Autodesk Fusion 360 part; units mm, degrees
sketch "Sketch1" plane through (0, 0, 0) normal (0, 0, 1) x (1, 0, 0) in component "Airfoil structure"
  spline S0 degree 5 poles (152.8506, 9.5306) (153.6754, 9.3537) (155.1958, 9.0287) (157.0885, 8.6275) (158.936, 8.2427) (160.6637, 7.8881) (162.4454, 7.5151) (164.8303, 6.998) (168.0437, 6.2836) (171.9513, 5.3996) (176.2204, 4.4167) (180.4193, 3.4264) (184.1364, 2.5129) (187.0894, 1.7283) (189.2467, 1.0645) (190.9412, 0.4268) (192.3181, -0.1665) (193.5665, -0.7111) (194.5238, -1.126) (195.0337, -1.3464) knots 0 0 0 0 0 0 0.066667 0.133333 0.2 0.266667 0.333333 0.4 0.466667 0.533333 0.6 0.666667 0.733333 0.8 0.866667 0.933333 1 1 1 1 1 1
  line L0 (148.4907, 10.4656) -> (157.2105, 8.5955)
  line L1 (191.9852, -0.0289) -> (198.0822, -2.6639)
  circle A0 centre (33.1388, 9.1296) radius 4.765
  circle A1 centre (116.1615, 7.0362) radius 3.175
  spline S1 degree 5 poles (-3.081, -1.3464) (-3.6016, -1.2536) (-4.5414, -1.0763) (-5.6463, -0.8353) (-6.5938, -0.5669) (-7.329, -0.2953) (-8.0513, 0.0089) (-9.0194, 0.5707) (-10.0683, 1.7874) (-10.9642, 3.2518) (-11.5103, 4.4866) (-11.5777, 5.0951) (-11.407, 5.643) (-11.0112, 6.6067) (-10.1307, 7.993) (-8.6022, 9.6431) (-6.4035, 11.272) (-4.1965, 12.5715) (-2.7349, 13.4061) (-1.8316, 13.8946) (-1.0216, 14.2664) (0.0955, 14.6934) (1.459, 15.1916) (2.6392, 15.6173) (3.2971, 15.8534) knots 0 0 0 0 0 0 0.05 0.1 0.15 0.2 0.25 0.3 0.35 0.4 0.45 0.5 0.55 0.6 0.65 0.7 0.75 0.8 0.85 0.9 0.95 1 1 1 1 1 1
  line L2 (0.5703, -1.9971) -> (-6.7323, -0.6957)
  line L3 (-0.0118, 14.6656) -> (6.606, 17.0412)
  line L4 (-8.4792, 9.8153) -> (-3.9569, 12.8132)
  line L5 (-11.5034, 4.2257) -> (-11.5345, 5.6935)
  line L6 (-7.2174, -0.5359) -> (-9.7443, 1.1286)
  line L7 (19.5688, 19.3646) -> (90.5688, 19.3646)
  spline S2 degree 5 poles (93.5688, 19.3646) (93.8188, 19.3387) (94.2829, 19.2905) (94.8714, 19.229) (95.4658, 19.1659) (96.0263, 19.1049) (96.567, 19.0445) (97.2368, 18.9678) (98.1315, 18.8622) (99.313, 18.7173) (100.8214, 18.5245) (102.3118, 18.3263) (103.5973, 18.1504) (104.53, 18.0207) (105.0153, 17.9528) knots 0 0 0 0 0 0 0.1 0.2 0.3 0.4 0.5 0.6 0.7 0.8 0.9 1 1 1 1 1 1
  line L8 (92.266, 19.4996) -> (94.8715, 19.2297)
  line L9 (103.6448, 18.1447) -> (106.3858, 17.761)
  spline S3 degree 5 poles (6.5765, 16.943) (6.9079, 17.0449) (7.5374, 17.2364) (8.3817, 17.4868) (9.3156, 17.7508) (10.2084, 17.9865) (10.8922, 18.156) (11.4504, 18.29) (11.9864, 18.4184) (12.6265, 18.5675) (13.504, 18.76) (14.4962, 18.9637) (15.447, 19.1503) (16.1786, 19.2906) (16.5688, 19.3646) knots 0 0 0 0 0 0 0.1 0.2 0.3 0.4 0.5 0.6 0.7 0.8 0.9 1 1 1 1 1 1
  line L10 (5.4107, 16.5846) -> (7.7424, 17.3015)
  line L11 (15.2328, 19.111) -> (17.9048, 19.6183)
  line L12 (152.4045, 9.626) -> (152.8506, 9.5306)
  line L13 (107.9851, 17.5282) -> (108.4359, 17.4637)
  line L14 (6.1441, 16.7993) -> (6.5765, 16.943)
  line L15 (128.8588, -1.3464) -> (132.3138, -1.3464)
  line L16 (149.471, 10.2539) -> (148.8431, 7.3203)
  line L17 (148.8431, 7.3203) -> (151.7767, 6.6925)
  line L18 (151.7767, 6.6925) -> (152.4045, 9.626)
  line L19 (3.2971, 15.8534) -> (4.243, 13.0064)
  line L20 (4.243, 13.0064) -> (7.09, 13.9524)
  line L21 (7.09, 13.9524) -> (6.1441, 16.7993)
  line L22 (160.8934, -1.3464) -> (160.8934, 1.6536)
  line L23 (160.8934, 1.6536) -> (163.8934, 1.6536)
  line L24 (163.8934, 1.6536) -> (163.8934, -1.3464)
  line L25 (132.3138, -1.3464) -> (160.8934, -1.3464)
  line L26 (163.8934, -1.3464) -> (195.0337, -1.3464)
  line L27 (3.4513, -1.3464) -> (3.4513, 1.6536)
  line L28 (3.4513, 1.6536) -> (6.4513, 1.6536)
  line L29 (6.4513, 1.6536) -> (6.4513, -1.3464)
  line L30 (-3.081, -1.3464) -> (3.4513, -1.3464)
  line L31 (6.4513, -1.3464) -> (128.8588, -1.3464)
  line L32 (105.0153, 17.9528) -> (107.9851, 17.5282)
  line L33 (19.5688, 19.3646) -> (19.5688, 16.3646)
  line L34 (19.5688, 16.3646) -> (16.5688, 16.3646)
  line L35 (16.5688, 16.3646) -> (16.5688, 19.3646)
  line L36 (90.5688, 19.3646) -> (90.5688, 16.3646)
  line L37 (90.5688, 16.3646) -> (93.5688, 16.3646)
  line L38 (93.5688, 16.3646) -> (93.5688, 19.3646)
  line L39 (113.7881, 13.5683) -> (110.8279, 14.0557)
  line L40 (110.8279, 14.0557) -> (111.3153, 17.0159)
  line L41 (113.7881, 13.5683) -> (114.2755, 16.5285)
  spline S4 degree 5 poles (108.4359, 17.4637) (108.6467, 17.433) (108.9931, 17.3831) (109.2865, 17.3426) (109.4547, 17.3194) (110.0313, 17.2264) (110.7239, 17.113) (111.2088, 17.0334) (111.3153, 17.0159) knots 0 0 0 0 0 0 0.066667 0.133333 0.2 0.217791 0.217791 0.217791 0.217791 0.217791 0.217791
  line L42 (107.9387, 17.5361) -> (108.933, 17.3913)
  line L43 (110.8712, 17.0888) -> (111.7595, 16.9429)
  spline S5 degree 5 poles (114.2755, 16.5285) (114.6969, 16.4591) (115.8472, 16.2695) (117.9388, 15.9249) (121.2621, 15.3773) (125.9027, 14.6124) (130.8234, 13.7994) (135.1309, 13.0827) (138.47, 12.5166) (140.7881, 12.1042) (142.4392, 11.78) (143.9897, 11.4433) (145.6466, 11.0766) (147.3521, 10.7068) (148.7253, 10.4127) (149.471, 10.2539) knots 0.291405 0.291405 0.291405 0.291405 0.291405 0.291405 0.333333 0.4 0.466667 0.533333 0.6 0.666667 0.733333 0.8 0.866667 0.933333 1 1 1 1 1 1
  line L44 (111.4536, 16.9935) -> (117.0973, 16.0636)
  line L45 (143.5745, 11.5101) -> (155.3674, 8.9976)
  point P0 (-8.4808, 0.2964)
  point P1 (-11.5189, 4.9596)
  point P2 (-6.2181, 11.3142)
  point P3 (11.4183, 18.2822)
  point P4 (96.5722, 19.0435)
  point P5 (109.7229, 17.2753)
  point P6 (137.8507, 12.6179)
  point P7 (163.7248, 7.2358)
  point P8 (186.791, 1.7868)
  dimension "d38" = 77
  dimension "d53" = 9.53
  dimension "d54" = 6.35
  dimension "d59" = 3
extrude "Extrude2" add sketch "Sketch1" along normal blind 3 contours S0 L0 L1 S1 L7 S2 L8 L9 S3 L12 L13 L14 L15 L16 L17 L18 L19 L20 L21 L22 L23 L24 L25 L26 L27 L28 L29 L30 L31 L32 L33 L34 L35 L36 L37 L38 L39 L40 L41 S4 L42 L43 S5 L44
sketch "lazercut" plane through (0, 0, 3) normal (0, 0, 1) x (1, 0, 0)
  circle A0 centre (33.1388, 9.1296) radius 4.765
  circle A1 centre (116.1615, 7.0362) radius 3.175
  line L0 (113.7881, 13.5683) -> (110.8279, 14.0557)
  line L1 (110.8279, 14.0557) -> (111.3153, 17.0159)
  spline S0 degree 5 poles (111.3153, 17.0159) (111.2088, 17.0334) (110.7239, 17.113) (110.0313, 17.2264) (109.4547, 17.3194) (109.2865, 17.3426) (108.9931, 17.3831) (108.6467, 17.433) (108.4359, 17.4637) knots -0.217791 -0.217791 -0.217791 -0.217791 -0.217791 -0.217791 -0.2 -0.133333 -0.066667 0 0 0 0 0 0
  line L2 (108.4359, 17.4637) -> (105.0153, 17.9528)
  spline S1 degree 5 poles (105.0153, 17.9528) (104.53, 18.0207) (103.5973, 18.1504) (102.3118, 18.3263) (100.8214, 18.5245) (99.313, 18.7173) (98.1315, 18.8622) (97.2368, 18.9678) (96.567, 19.0445) (96.0263, 19.1049) (95.4658, 19.1659) (94.8714, 19.229) (94.2829, 19.2905) (93.8188, 19.3387) (93.5688, 19.3646) knots -1 -1 -1 -1 -1 -1 -0.9 -0.8 -0.7 -0.6 -0.5 -0.4 -0.3 -0.2 -0.1 0 0 0 0 0 0
  line L3 (93.5688, 19.3646) -> (93.5688, 16.3646)
  line L4 (93.5688, 16.3646) -> (90.5688, 16.3646)
  line L5 (90.5688, 16.3646) -> (90.5688, 19.3646)
  line L6 (90.5688, 19.3646) -> (19.5688, 19.3646)
  line L7 (19.5688, 19.3646) -> (19.5688, 16.3646)
  line L8 (19.5688, 16.3646) -> (16.5688, 16.3646)
  line L9 (16.5688, 16.3646) -> (16.5688, 19.3646)
  spline S2 degree 5 poles (16.5688, 19.3646) (16.1786, 19.2906) (15.447, 19.1503) (14.4962, 18.9637) (13.504, 18.76) (12.6265, 18.5675) (11.9864, 18.4184) (11.4504, 18.29) (10.8922, 18.156) (10.2084, 17.9865) (9.3156, 17.7508) (8.3817, 17.4868) (7.5374, 17.2364) (6.9079, 17.0449) (6.5765, 16.943) knots -1 -1 -1 -1 -1 -1 -0.9 -0.8 -0.7 -0.6 -0.5 -0.4 -0.3 -0.2 -0.1 0 0 0 0 0 0
  line L10 (6.5765, 16.943) -> (6.1441, 16.7993)
  line L11 (6.1441, 16.7993) -> (7.09, 13.9524)
  line L12 (7.09, 13.9524) -> (4.243, 13.0064)
  line L13 (4.243, 13.0064) -> (3.2971, 15.8534)
  spline S3 degree 5 poles (3.2971, 15.8534) (2.6392, 15.6173) (1.459, 15.1916) (0.0955, 14.6934) (-1.0216, 14.2664) (-1.8316, 13.8946) (-2.7349, 13.4061) (-4.1965, 12.5715) (-6.4035, 11.272) (-8.6022, 9.6431) (-10.1307, 7.993) (-11.0112, 6.6067) (-11.407, 5.643) (-11.5777, 5.0951) (-11.5103, 4.4866) (-10.9642, 3.2518) (-10.0683, 1.7874) (-9.0194, 0.5707) (-8.0513, 0.0089) (-7.329, -0.2953) (-6.5938, -0.5669) (-5.6463, -0.8353) (-4.5414, -1.0763) (-3.6016, -1.2536) (-3.081, -1.3464) knots -1 -1 -1 -1 -1 -1 -0.95 -0.9 -0.85 -0.8 -0.75 -0.7 -0.65 -0.6 -0.55 -0.5 -0.45 -0.4 -0.35 -0.3 -0.25 -0.2 -0.15 -0.1 -0.05 0 0 0 0 0 0
  line L14 (-3.081, -1.3464) -> (3.4513, -1.3464)
  line L15 (3.4513, -1.3464) -> (3.4513, 1.6536)
  line L16 (3.4513, 1.6536) -> (6.4513, 1.6536)
  line L17 (6.4513, 1.6536) -> (6.4513, -1.3464)
  line L18 (6.4513, -1.3464) -> (160.8934, -1.3464)
  line L19 (160.8934, -1.3464) -> (160.8934, 1.6536)
  line L20 (160.8934, 1.6536) -> (163.8934, 1.6536)
  line L21 (163.8934, 1.6536) -> (163.8934, -1.3464)
  line L22 (163.8934, -1.3464) -> (195.0337, -1.3464)
  spline S4 degree 5 poles (195.0337, -1.3464) (194.5238, -1.126) (193.5665, -0.7111) (192.3181, -0.1665) (190.9412, 0.4268) (189.2467, 1.0645) (187.0894, 1.7283) (184.1364, 2.5129) (180.4193, 3.4264) (176.2204, 4.4167) (171.9513, 5.3996) (168.0437, 6.2836) (164.8303, 6.998) (162.4454, 7.5151) (160.6637, 7.8881) (158.936, 8.2427) (157.0885, 8.6275) (155.1958, 9.0287) (153.6754, 9.3537) (152.8506, 9.5306) knots -1 -1 -1 -1 -1 -1 -0.933333 -0.866667 -0.8 -0.733333 -0.666667 -0.6 -0.533333 -0.466667 -0.4 -0.333333 -0.266667 -0.2 -0.133333 -0.066667 0 0 0 0 0 0
  line L23 (152.8506, 9.5306) -> (152.4045, 9.626)
  line L24 (152.4045, 9.626) -> (151.7767, 6.6925)
  line L25 (151.7767, 6.6925) -> (148.8431, 7.3203)
  line L26 (148.8431, 7.3203) -> (149.471, 10.2539)
  spline S5 degree 5 poles (149.471, 10.2539) (148.7253, 10.4127) (147.3521, 10.7068) (145.6466, 11.0766) (143.9897, 11.4433) (142.4392, 11.78) (140.7881, 12.1042) (138.47, 12.5166) (135.1309, 13.0827) (130.8234, 13.7994) (125.9027, 14.6124) (121.2621, 15.3773) (117.9388, 15.9249) (115.8472, 16.2695) (114.6969, 16.4591) (114.2755, 16.5285) knots -1 -1 -1 -1 -1 -1 -0.933333 -0.866667 -0.8 -0.733333 -0.666667 -0.6 -0.533333 -0.466667 -0.4 -0.333333 -0.291405 -0.291405 -0.291405 -0.291405 -0.291405 -0.291405
  line L27 (114.2755, 16.5285) -> (113.7881, 13.5683)
sketch "Sketch3" plane through (0, 0, 0) normal (0, 0, 1) x (1, 0, 0)
component "Airfoil structure" placed x (1, 0, 0) y (0, 1, 0) z (0, 0, 1) at (0, 0, 0)
Could you check a few things on this model? Use its own coordinates, in mm. Round coordinates to 2 decimals unless told otherwise and drop trailing zeros.
(1) I'm going to push flat-ended pins straight in: pin 1 (7.5 mm diameter, centred on x = 33.14, y = 9.13, fed in from +Z); pin 2 (0.9 mm diameter, centred on y = 0, z = 1, fed in from +X); pin 3 (0.9 mm diameter, centred on x = 18.5, z = 1, fed in from +Y). Where does each tip first touch, or does it pass through?
Response values:
pin 1: passes through
pin 2: stops at x = 192.97
pin 3: stops at y = 16.36
(2) Imagine slicing it at A-A (z = 1.7). Count the separate pieces of the cut face and the enclosed holes in it, plus the area to 3 significant figures.
Response values:
separate pieces: 1
enclosed holes: 2
area: 3,090 mm2
(3) Please list where these lines run through material, in increasing order: line 1 along X through (y, z) = (9.75, 1.5); line 2 along Y through (x, z) = (17, 0.2); line 3 along Y through (x, z) = (34.5, 0.9).
Response values:
line 1: x = -8.31 to 28.41, 37.86 to 114.51, 117.81 to 149.36
line 2: y = -1.35 to 16.36
line 3: y = -1.35 to 4.56, 13.7 to 19.36
